from build123d import *

# Parameters (mm, degrees)
EXTRUDE_1_DEPTH     = 8
SKETCH_2_R          = 5
SKETCH_2_R_2        = 2
SKETCH_2_R_3        = 9.5
CUT_EXTRUDE_1_DEPTH = 8
SKETCH_3_W          = 21
SKETCH_3_H          = 40.5
CUT_EXTRUDE_2_DEPTH = 10
SKETCH_4_R          = 1.5
CUT_EXTRUDE_3_DEPTH = 10
SKETCH_5_R          = 1
CUT_EXTRUDE_4_DEPTH = 10
SKETCH_6_W          = 18
SKETCH_6_H          = 50
CUT_EXTRUDE_5_DEPTH = 10


with BuildPart() as part:
    # 草图1 → 凸台-拉伸1 (new body)
    with BuildSketch(Plane.XY):
        with BuildLine():
            ThreePointArc((13, 80.516685226), (0, 73), (-13, 80.516685226))
            Line((-13, 80.516685226), (-13, -80.516685226))
            ThreePointArc((-13, -80.516685226), (0, -73), (13, -80.516685226))
            Line((13, -80.516685226), (13, 80.516685226))
        make_face()
        with BuildLine():
            Line((-13, 80.516685226), (-13, 88))
            Line((-13, 88), (13, 88))
            Line((13, 88), (13, 80.516685226))
            ThreePointArc((13, 80.516685226), (14.491376746, 84.127016654), (15, 88))
            ThreePointArc((15, 88), (-3.872983346, 102.491376746), (-13, 80.516685226))
        make_face()
        with BuildLine():
            Line((13, 88), (-13, 88))
            Line((-13, 88), (-13, 80.516685226))
            ThreePointArc((-13, 80.516685226), (0, 73), (13, 80.516685226))
            Line((13, 80.516685226), (13, 88))
        make_face()
        with BuildLine():
            ThreePointArc((13, -80.516685226), (0, -73), (-13, -80.516685226))
            Line((-13, -80.516685226), (-13, -88))
            Line((-13, -88), (13, -88))
            Line((13, -88), (13, -80.516685226))
        make_face()
        with BuildLine():
            Line((-13, -88), (-13, -80.516685226))
            ThreePointArc((-13, -80.516685226), (-3.872983346, -102.491376746), (15, -88))
            ThreePointArc((15, -88), (14.491376746, -84.127016654), (13, -80.516685226))
            Line((13, -80.516685226), (13, -88))
            Line((13, -88), (-13, -88))
        make_face()
    extrude(amount=EXTRUDE_1_DEPTH)

    # 草图2 → 切除-拉伸1 (cut)
    with BuildSketch(Plane.XY.offset(8)):
        with Locations((0, 88)):
            Circle(SKETCH_2_R)
        with Locations((0, 98)):
            Circle(SKETCH_2_R_2)
        with Locations((10, 88)):
            Circle(SKETCH_2_R_2)
        with Locations((0, 78)):
            Circle(SKETCH_2_R_2)
        with Locations((-10, 88)):
            Circle(SKETCH_2_R_2)
        with Locations((0, -88)):
            Circle(SKETCH_2_R_3)
        with Locations((7.071067812, 95.071067812)):
            Circle(SKETCH_2_R_2)
        with Locations((7.071067812, 80.928932188)):
            Circle(SKETCH_2_R_2)
        with Locations((-7.071067812, 80.928932188)):
            Circle(SKETCH_2_R_2)
        with Locations((-7.071067812, 95.071067812)):
            Circle(SKETCH_2_R_2)
    extrude(amount=-CUT_EXTRUDE_1_DEPTH, mode=Mode.SUBTRACT)

    # 草图3 → 切除-拉伸2 (cut)
    with BuildSketch(Plane.XY.offset(8)):
        with Locations((0, -40.25)):
            Rectangle(SKETCH_3_W, SKETCH_3_H)
    extrude(amount=-CUT_EXTRUDE_2_DEPTH, mode=Mode.SUBTRACT)

    # 草图4 → 切除-拉伸3 (cut)
    with BuildSketch(Plane.XY.offset(8)):
        with Locations((-5, -16)):
            Circle(SKETCH_4_R)
        with Locations((5, -16)):
            Circle(SKETCH_4_R)
        with Locations((-5, -64.5)):
            Circle(SKETCH_4_R)
        with Locations((5, -64.5)):
            Circle(SKETCH_4_R)
    extrude(amount=-CUT_EXTRUDE_3_DEPTH, mode=Mode.SUBTRACT)

    # 草图5 → 切除-拉伸4 (cut)
    with BuildSketch(Plane.XY.offset(8)):
        with Locations((-9.5, -20)):
            Circle(SKETCH_5_R)
        with Locations((9.5, -20)):
            Circle(SKETCH_5_R)
        with Locations((9.5, -60.5)):
            Circle(SKETCH_5_R)
        with Locations((-9.5, -60.5)):
            Circle(SKETCH_5_R)
    extrude(amount=-CUT_EXTRUDE_4_DEPTH, mode=Mode.SUBTRACT)

    # 草图6 → 切除-拉伸5 (cut)
    with BuildSketch(Plane.XY.offset(8)):
        with BuildLine():
            ThreePointArc((-9, 54.75), (0, 63.75), (9, 54.75))
            Line((9, 54.75), (-9, 54.75))
        make_face()
        with Locations((0, 29.75)):
            Rectangle(SKETCH_6_W, SKETCH_6_H)
        with BuildLine():
            Line((-9, 4.75), (9, 4.75))
            ThreePointArc((9, 4.75), (0, -4.25), (-9, 4.75))
        make_face()
    extrude(amount=-CUT_EXTRUDE_5_DEPTH, mode=Mode.SUBTRACT)


solid = part.part
Can you work these out from the model? Positions are in its coordinate system, mm. A direction names the side the tool comes from. Round coordinates to 2 decimals unless told otherwise and drop trailing zeros. Loops run counter-clockwise (first coordinate to the right, second up) from the corner with the lowest first, then second, coordinate; pieces in that order, holes last. Notation, with made-up numbers: (36, 16) - (40, 16) arc R16 ccw to (40, 20) - close; hole circle Ø9 at (6.25, -7). An arc over 180 degrees is marked (long way). Answer in a Markdown table with one row per item. Add a question column.
Q1. Which directions (+Z, -Z, +X, -X, +Y, -Y) give clear straight access to the entire face, cutting with the end or side of a thin tool? Please do faces 3 (the flat face through (-10, 24, 8)), 4 (the cylindrical face through (-0.198, 63.748, 4.056)).
Q2. I need wall thicknesses on L1, parallel to X at y = -64.5, z = 2.25; L2, parallel to X at y = -55, z = 3.25; L3, parallel to X at y = 5, z = 5.25. Which ranges of each line are inside material? Lowest first, please.
Q3. I want a section at B-B on z = 6. Count the separate pieces of the cut face and the enclosed holes in it, and give its area (3 significant figures).
Q4. I want a section at D-D on y = 0.5. List the corners of the cut face in (x, z) for me, and give its area (3 significant figures).
Q5. I want a section at C-C on y = 66.5. List the corners of the cut face in (x, z) for me, and give its area (3 significant figures).
Q6. For pin 1 Ø1.5 at (x, z) = (-10.5, 4) entering from +Y; pin 2 Ø1.5 at (y, z) = (73.5, 7) entering from -X; pin 3 Ø2 at (x, z) = (3, 7) entering from +Y, each with a flat end and sliding along its axis, tell me the tip position at first contact or that it passes through.
Q7. We'd pull the mould along Y, two halves only. Please class faces 1 (the flat face through (0, -20, 4)), 2 (the flat face through (-10, 24, 0)): pulls with the +Y half, pulls with the -Y half, needs draft (parallel to the pull), parting line crosses it, or undercut.
Q8. I want a section at A-A on y = -34. List the corners of the cut face in (x, z) for me.
A:
| question | item | result |
|---|---|---|
| 1 | face 3 | +Z, +X, -X, +Y, -Y |
| 1 | face 4 | +Z, -Z |
| 2 | L1 | -13 to -6.5, -3.5 to 3.5, 6.5 to 13 |
| 2 | L2 | -13 to -10.5, 10.5 to 13 |
| 2 | L3 | -13 to -9, 9 to 13 |
| 3 | separate pieces | 1 |
| 3 | enclosed holes | 16 |
| 3 | area | 2,820 mm^2 |
| 4 | outline | (-13, 0) - (-7.93, 0) - (-7.93, 8) - (-13, 8) - close; (7.93, 0) - (13, 0) - (13, 8) - (7.93, 8) - close |
| 4 | area | 81.1 mm^2 |
| 5 | outline | (-13, 0) - (13, 0) - (13, 8) - (-13, 8) - close |
| 5 | area | 208 mm^2 |
| 6 | pin 1 | y = 99.4 |
| 6 | pin 2 | x = -13 |
| 6 | pin 3 | y = 102.87 |
| 7 | face 1 | undercut |
| 7 | face 2 | needs draft |
| 8 | outline | (-13, 0) - (-10.5, 0) - (-10.5, 8) - (-13, 8) - close; (10.5, 0) - (13, 0) - (13, 8) - (10.5, 8) - close |
